```python
from build123d import *

# Parameters (mm, degrees)
SKETCH1_R           = 1.75
BOSS_EXTRUDE1_DEPTH = 4


with BuildPart() as part:
    # Sketch1 → Boss-Extrude1 (new body)
    with BuildSketch(Plane.XY):
        with BuildLine():
            Line((2023.821699886, 391.448846192), (2023.821699886, -18.551153808))
            Line((2023.821699886, -18.551153808), (1864.321699886, -18.551153808))
            ThreePointArc((1864.321699886, -18.551153808), (1825.430826921, -2.442026773), (1809.321699886, 36.448846192))
            Line((1809.321699886, 36.448846192), (1809.321699886, 336.448846192))
            ThreePointArc((1809.321699886, 336.448846192), (1825.430826921, 375.339719157), (1864.321699886, 391.448846192))
            Line((1864.321699886, 391.448846192), (2023.821699886, 391.448846192))
        make_face()
        with Locations((2012.76292798, -11.051153808)):
            Circle(SKETCH1_R, mode=Mode.SUBTRACT)
        with Locations((1864.321699886, -11.051153808)):
            Circle(SKETCH1_R, mode=Mode.SUBTRACT)
        with Locations((1816.821699886, 36.448846192)):
            Circle(SKETCH1_R, mode=Mode.SUBTRACT)
        with Locations((1816.821699886, 186.448846192)):
            Circle(SKETCH1_R, mode=Mode.SUBTRACT)
        with Locations((1816.821699886, 336.448846192)):
            Circle(SKETCH1_R, mode=Mode.SUBTRACT)
        with Locations((1864.321699886, 383.948846192)):
            Circle(SKETCH1_R, mode=Mode.SUBTRACT)
        with Locations((2012.76292798, 383.948846192)):
            Circle(SKETCH1_R, mode=Mode.SUBTRACT)
    extrude(amount=BOSS_EXTRUDE1_DEPTH)


solid = part.part
```
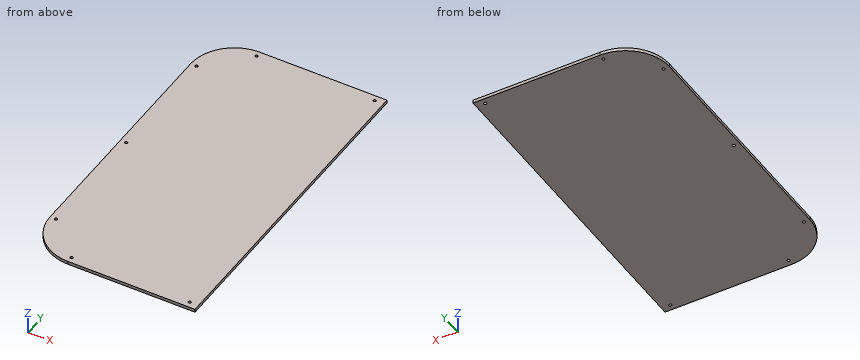
The model under review builds one solid part; all positions refer to its coordinate system, in mm. Coordinates: 2 decimals unless noted, no trailing zeros. Write each loop counter-clockwise with the first axis right and the second up, starting at its lowest first coordinate (ties: lowest second). Pieces come first, ordered by that corner, then holes. Notation, with made-up numbers: (-38.5, 8.5) -> (9.5, 8.5) arc R27 cw to (9.5, 38.5) -> close; hole circle Ø1 at (34, -7). An arc over 180 degrees is marked (long way). One line per item, written item: value. Start each with the question number.
Q1. To check wall thickness, follow probe 1 along Y at (x, z) = (1863.5, 2.6); probe 2 along X at (y, z) = (4, 3.6); probe 3 along X at (y, z) = (359.5, 1.6). State the ranges of each line that lie inside material, in increasing order.
Q2. Add section C-C, the plane x = 1839. Give the boundary of the cut face in (y, z).
Q3. Clearance check with a flat-ended pin moving along its axis: P1, Ø3, axis at x = 2012.76, y = -11.05, coming from the +Z side. State where the tip first meets the part, or that it passes through.
Q4. Add section A-A, the plane z = 0.7. Give the boundary of the cut face in (x, y), then the cut area to 3 significant figures.
Q5. Add section B-B, the plane y = 363.5. Give the boundary of the cut face in (x, z), then the cut area to 3 significant figures.
Response:
1. probe 1: -18.55 to -12.6, -9.51 to 382.4, 385.49 to 391.44
1. probe 2: 1819.91 to 2023.82
1. probe 3: 1814.39 to 2023.82
2. outline: (-12.38, 0) -> (385.27, 0) -> (385.27, 4) -> (-12.38, 4) -> close
3. P1: through
4. outline: (1809.32, 36.45) arc R55 ccw to (1864.32, -18.55) -> (2023.82, -18.55) -> (2023.82, 391.45) -> (1864.32, 391.45) arc R55 ccw to (1809.32, 336.45) -> close; hole circle Ø3.5 at (1816.82, 36.45); hole circle Ø3.5 at (1816.82, 186.45); hole circle Ø3.5 at (1816.82, 336.45); hole circle Ø3.5 at (1864.32, -11.05); hole circle Ø3.5 at (1864.32, 383.95); hole circle Ø3.5 at (2012.76, -11.05); hole circle Ø3.5 at (2012.76, 383.95)
4. area: 86,600 mm²
5. outline: (1816.43, 0) -> (2023.82, 0) -> (2023.82, 4) -> (1816.43, 4) -> close
5. area: 830 mm²
